For this review, use the dimensioned drawing (mm, ordinates from the lowest corner) and the shaded views. A direction names the side the tool comes from. Coordinates: 2 decimals unless noted, no trailing zeros. Order: outer loops, then holes, each group sorted by start corner. A loop starts at its lowest first (then second) coordinate and runs counter-clockwise, first axis right, second up. Notation, with made-up numbers: (14, 65.5) -> (43, 65.5) arc R20 cw to (43, 100.5) -> close; hole circle Ø9 at (52.25, 10). An arc over 180 degrees is marked (long way). Return JSON: item names as keys, results as strings. Group by question number.
Item 1: Take a section at D-D (z = 7.5). Write out the cut boundary in (x, y) (1 decimal), then the cut area to 3 significant figures.
Item 2: Draft analysis for pull direction X (two halves, no side actions). For the marked faces 3, 4 and 5, state which applies: +X half, -X half, draft (parallel to the pull), parting line (faces both ways), or undercut.
Item 3: Machinability: for the marked faces 1 and 2, which of the approach directions +Z, -Z, +X, -X, +Y, -Y give a long, thin tool a straight path to every point of the face, cutting with its end or side? Answer none if there is none.
Item 4: Insertion check: pin 1 (3 mm diameter, centred on y = 39, z = 7.5, fed in from -X); pin 2 (2 mm diameter, centred on y = 6, z = 3.5, fed in from -X); pin 3 (5 mm diameter, centred on y = 13, z = 9, fed in from -X). Each pin has a flat end and moves straight along its axis. Give the tip position at first contact, or say it passes through.
Item 5: For line 1 along X through (y, z) = (20.5, 2.25) (1 decimal); line 2 along X through (y, z) = (24.5, 7.25) (1 decimal); line 3 along Z through (x, y) = (35, 7), list the stretches that pass through material, from the lowest coordinate up.
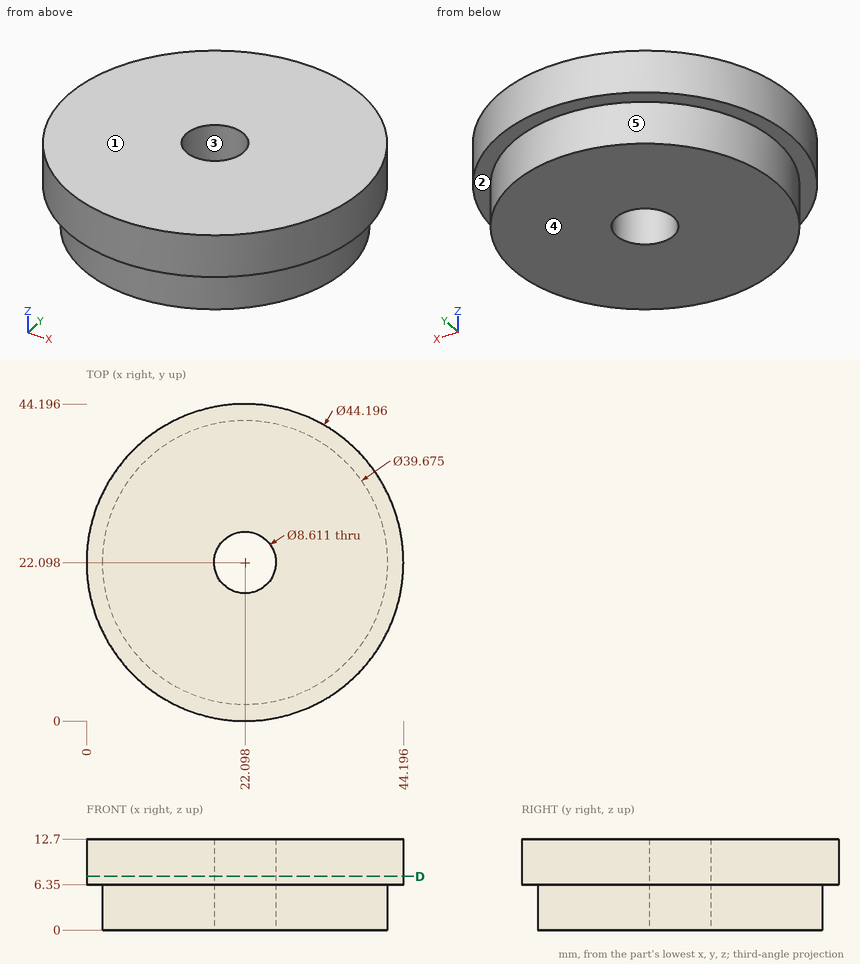
Findings below:
{
 "1": {"outline": "circle Ø44.2 at (22.1, 22.1); hole circle Ø8.6 at (22.1, 22.1)", "area": "1,480 mm2"},
 "2": {"face 3": "undercut", "face 4": "draft", "face 5": "parting line"},
 "3": {"face 1": "+Z, +X, -X, +Y, -Y", "face 2": "-Z"},
 "4": {"pin 1": "stops at x = 6.25", "pin 2": "stops at x = 9.23", "pin 3": "stops at x = 1.01"},
 "5": {"line 1": "x = 2.3 to 18.1, 26.1 to 41.9", "line 2": "x = 0.1 to 18.5, 25.7 to 44.1", "line 3": "z = 6.35 to 12.7"}
}
